The listing builds one solid part. Answer for the finished solid, in the listing's coordinates (mm). Face numbers are marked on the shaded views. Give positions to 0.01 mm unless a question says otherwise; leave off trailing zeros. Order: outer loops, then holes, each group sorted by start corner. A loop starts at its lowest first (then second) coordinate and runs counter-clockwise, first axis right, second up.
Autodesk Inventor part; units mm, degrees
ref_plane "YZ Plane" through (0, 0, 0) normal (1, 0, 0) x (0, 1, 0)
ref_plane "XZ Plane" through (0, 0, 0) normal (0, 1, 0) x (-1, 0, 0)
ref_plane "XY Plane" through (0, 0, 0) normal (0, 0, 1) x (1, 0, 0)
sketch "Sketch1" plane through (0, 0, 0) normal (0, 1, 0) x (-1, 0, 0)
  circle A0 centre (0, 0) radius 3.175
  dimension "d0" = 6.35
extrude "Extrusion1" add sketch "Sketch1" along normal blind 44.45
sketch "Sketch2" plane through (0, 44.45, 0) normal (0, 1, 0) x (1, 0, 0)
  circle A0 centre (0, 0) radius 3.175
  circle A1 centre (0, 0) radius 4.7625
  dimension "d3" = 9.525
extrude "Extrusion2" add sketch "Sketch2" along normal blind 6.35 contours A0 | A1
sketch "Sketch3" plane through (0, 50.8, 0) normal (0, 1, 0) x (1, 0, 0)
  circle A0 centre (0, 0) radius 4.7625
  line L0 (-1.3748, 2.3812) -> (1.3748, 2.3813)
  line L1 (1.3748, 2.3813) -> (2.7496, 0)
  line L2 (2.7496, 0) -> (1.3748, -2.3813)
  line L3 (1.3748, -2.3813) -> (-1.3748, -2.3813)
  line L4 (-1.3748, -2.3813) -> (-2.7496, 0)
  line L5 (-2.7496, 0) -> (-1.3748, 2.3812)
  dimension "d6" = 4.7625
extrude "Extrusion3" cut sketch "Sketch3" against normal blind 3.175 contours L0 L1 L2 L3 L4 L5
fillet "Fillet1" radius 0.3969 3 edges at (3.175, 44.45, 0) (-4.7625, 50.8, 0) (3.175, 0, 0)
properties part number "Bolt_0.25_20_1.75len_SocketHead" material "Stainless Steel, Austenitic"
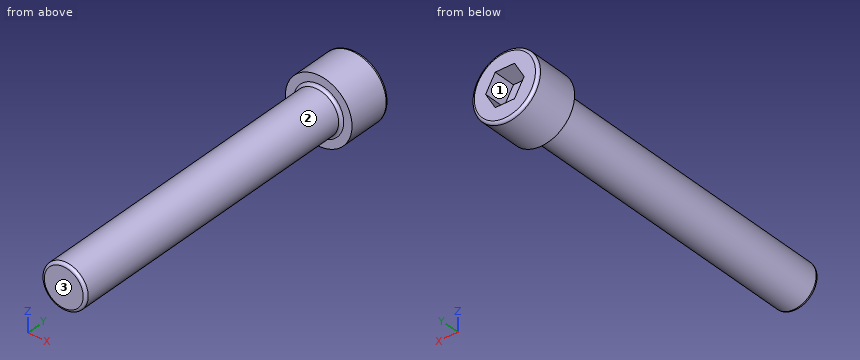
1) Find section C-C (y = 47). Write down the section's boundary in (x, z) (1 decimal).
Geometry says:
outline: circle Ø9.5 at (0, 0)
2) Find section A-A (y = 6.5). Write down the section's boundary in (x, z) (3 decimals), then the cut area to 3 significant figures.
Geometry says:
outline: circle Ø6.35 at (0, 0)
area: 31.7 mm2
3) For a pull along Z with two mould halves and no side action, classify the marked faces 1, 2 and 3 as +Z half, -Z half, draft (parallel to the pull), parting line (faces both ways), or undercut.
Geometry says:
face 1: undercut
face 2: parting line
face 3: draft
4) Straight lines are drawn through the part: probe 1 along Y at (x, z) = (-0.5, 1) (3 decimals); probe 2 along Y at (x, z) = (-2.25, 3); probe 3 along X at (y, z) = (18.5, 0.25). For each, find the intervals that lie inside material, in ascending order.
Geometry says:
probe 1: y = 0 to 47.625
probe 2: y = 44.45 to 50.8
probe 3: x = -3.17 to 3.17
5) Given P1, Ø1.4, axis at x = 0.5, z = 0, coming from the +Y side (3 decimals); P2, Ø3, axis at y = 22, z = 0.5, coming from the +X side (3 decimals); P3, Ø1, axis at y = 10, z = 1, coming from the -X side, each flat-ended and moving along its own axis, determine where each tip first touches the part or whether it passes through.
Geometry says:
P1: stops at y = 47.625
P2: stops at x = 3.175
P3: stops at x = -3.14
